Autodesk Inventor part; units mm, degrees
ref_plane "YZ Plane" through (0, 0, 0) normal (1, 0, 0) x (0, 1, 0)
ref_plane "XZ Plane" through (0, 0, 0) normal (0, 1, 0) x (-1, 0, 0)
ref_plane "XY Plane" through (0, 0, 0) normal (0, 0, 1) x (1, 0, 0)
sketch "Sketch1" plane through (0, 0, 0) normal (0, 0, 1) x (1, 0, 0)
  line L0 (0, 0) -> (0, 5.75)
  line L1 (0, 5.75) -> (3, 5.75)
  line L2 (3, 5.75) -> (3, 6.75)
  line L3 (20.9195, 5.0497) -> (20.9195, 0.95)
  line L4 (20.9195, 0.95) -> (32.6195, 0.95)
  line L5 (33.1195, 0.45) -> (33.1195, 0)
  line L6 (33.1195, 0) -> (0, 0)
  arc A0 (33.1195, 0.45) -> (32.6195, 0.95) centre (32.6195, 0.45) ccw
  line L7 (-7.1846, 0) -> (0, 0) construction
  line L8 (3, 6.75) -> (11.155, 6.4559)
  line L9 (11.155, 6.4559) -> (20.9195, 5.0497)
  point P0 (33.1195, 0.95)
  dimension "d0" = 5.75
  dimension "d1" = 3
  dimension "d2" = 1
  dimension "d3" = 18
  dimension "d5" = 12.2
  dimension "d6" = 0.5
  dimension "d11" = 0.95
revolve "Revolution1" add sketch "Sketch1" angle 360 about axis through (-7.1846, 0, 0) along (1, 0, 0)
sketch "Sketch2" plane through (0, 0, 0) normal (-1, 0, 0) x (0, 0, 1)
  circle A0 centre (0, 0) radius 2
  dimension "d8" = 4
extrude "Extrusion1" cut sketch "Sketch2" against normal blind 20
sketch "Sketch3" plane through (20.9195, 0, 0) normal (1, 0, 0) x (0, 0, -1)
  circle A0 centre (0, 0) radius 0.45
  circle A1 centre (0, 0) radius 2
  circle A2 centre (0, 0) radius 0.95
  circle A3 centre (0, 0) radius 0.95
  dimension "d12" = 4
extrude "Extrusion2" cut sketch "Sketch3" against normal blind 0.1 contours A1
properties part number "CT3149-0-Banana-Connector"
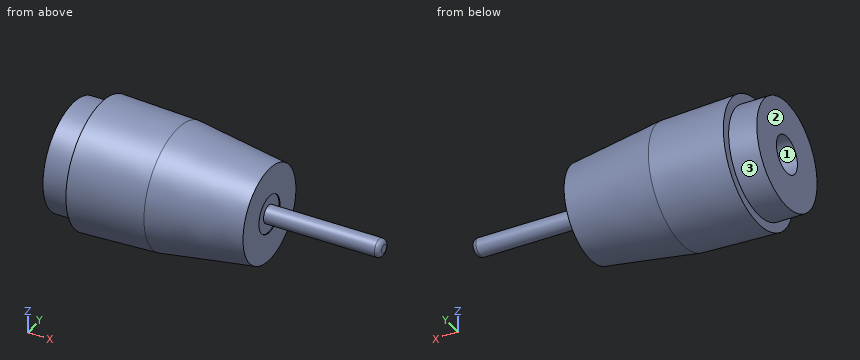
The listing builds one solid part. Answer for the finished solid, in the listing's coordinates (mm). Face numbers are marked on the shaded views. Coordinates: 2 decimals unless noted, no trailing zeros. Loops run counter-clockwise (first coordinate to the right, second up) from the corner with the lowest first, then second, coordinate; pieces in that order, holes last. Notation, with made-up numbers: (32, 44) - (38, 44) arc R22 ccw to (38, 67) - close; hole circle Ø11 at (68, 30). An arc over 180 degrees is marked (long way). Use a Markdown table: item, result. Add a question column.
1) The part is cut by section A-A, the plane x = 2.5. Give the vertices of the cut face in (y, z), and give its area (3 significant figures).
2) The part is cut by section B-B, the plane x = 28.5. Give the vertices of the cut face in (y, z), and give its area (3 significant figures).
3) The mould has two halves that part along Z. Classify the marked faces 1, 2 and 3: released by +Z, released by -Z, zero draft, split by the parting line, or undercut.
4) Given pin 1 (1.5 mm diameter, centred on x = 6.5, y = 2, fed in from -Z); pin 2 (3 mm diameter, centred on y = 0, z = 0, fed in from -X); pin 3 (2 mm diameter, centred on x = 10.5, z = 4.5, fed in from -Y), each flat-ended and moving along its own axis, determine where each tip first touches the part or whether it passes through.
5) Find the intervals of material crossed by line 1 (Z direction, x = 20.95, y = 0); line 2 (Y direction, x = 20.85, z = 0); line 3 (Z direction, x = 4, y = 1), in increasing order.
6) The part is cut by section C-C, the plane x = 19. Give the vertices of the cut face in (y, z), and give its area (3 significant figures).
Here are the results:
| question | item | result |
|---|---|---|
| 1 | outline | circle Ø11.5 at (0, 0); hole circle Ø4 at (0, 0) |
| 1 | area | 91.3 mm^2 |
| 2 | outline | circle Ø1.9 at (0, 0) |
| 2 | area | 2.84 mm^2 |
| 3 | face 1 | undercut |
| 3 | face 2 | zero draft |
| 3 | face 3 | split by the parting line |
| 4 | pin 1 | stops at z = -6.51 |
| 4 | pin 2 | stops at x = 20 |
| 4 | pin 3 | stops at y = -5.45 |
| 5 | line 1 | z = -0.95 to 0.95 |
| 5 | line 2 | y = -5.06 to -2, -0.95 to 0.95, 2 to 5.06 |
| 5 | line 3 | z = -6.64 to -1.73, 1.73 to 6.64 |
| 6 | outline | circle Ø10.65 at (0, 0); hole circle Ø4 at (0, 0) |
| 6 | area | 76.6 mm^2 |
